```python
from build123d import *

# Parameters (mm, degrees)
EXTRUDE_1_DEPTH     = 3
SKETCH_3_R          = 1.5
CUT_EXTRUDE_1_DEPTH = 3


with BuildPart() as part:
    # 草图2 → 凸台-拉伸1 (new body)
    with BuildSketch(Plane(origin=(0, 0, 0), x_dir=(0, 0, -1), z_dir=(1, 0, 0))):
        with BuildLine():
            Line((0, 0), (0, -15))
            Line((0, -15), (20, -15))
            Line((20, -15), (50, -15))
            Line((50, -15), (70, -15))
            Line((70, -15), (70, 0))
            Line((70, 0), (62.603277808, 0))
            ThreePointArc((62.603277808, 0), (60.294225904, 0.565106619), (58.507118205, 2.132688278))
            Line((58.507118205, 2.132688278), (43.403840397, 23.708799432))
            ThreePointArc((43.403840397, 23.708799432), (42.731310557, 25.07291423), (42.5, 26.576111154))
            Line((42.5, 26.576111154), (42.5, 35))
            Line((42.5, 35), (27.5, 35))
            Line((27.5, 35), (27.5, 26.576111154))
            ThreePointArc((27.5, 26.576111154), (27.268689443, 25.07291423), (26.596159603, 23.708799432))
            Line((26.596159603, 23.708799432), (11.492881795, 2.132688278))
            ThreePointArc((11.492881795, 2.132688278), (9.705774096, 0.565106619), (7.396722192, 0))
            Line((7.396722192, 0), (0, 0))
        make_face()
        with BuildLine():
            Line((22.877485177, -6.367544468), (23.86037961, -3.41886117))
            ThreePointArc((23.86037961, -3.41886117), (25.680244677, -0.943789074), (28.6037961, 0))
            Line((28.6037961, 0), (41.3962039, 0))
            ThreePointArc((41.3962039, 0), (44.319755323, -0.943789074), (46.13962039, -3.41886117))
            Line((46.13962039, -3.41886117), (47.122514823, -6.367544468))
            ThreePointArc((47.122514823, -6.367544468), (46.847632597, -8.169420569), (45.225148227, -9))
            Line((45.225148227, -9), (24.774851773, -9))
            ThreePointArc((24.774851773, -9), (23.152367403, -8.169420569), (22.877485177, -6.367544468))
        make_face(mode=Mode.SUBTRACT)
        with BuildLine():
            Line((29.256242147, 6), (31.5, 6))
            Line((31.5, 6), (31.5, 11))
            ThreePointArc((31.5, 11), (30.914213562, 12.414213562), (29.5, 13))
            Line((29.5, 13), (24.673666452, 13))
            ThreePointArc((24.673666452, 13), (25.072942015, 8.261387212), (29.256242147, 6))
        make_face(mode=Mode.SUBTRACT)
        with BuildLine():
            Line((30.57750685, 21.867311722), (29.256242147, 19))
            Line((29.256242147, 19), (40.091090757, 19))
            Line((40.091090757, 19), (38.769826055, 21.867311722))
            ThreePointArc((38.769826055, 21.867311722), (34.673666452, 24), (30.57750685, 21.867311722))
        make_face(mode=Mode.SUBTRACT)
        with BuildLine():
            Line((38.5, 11), (38.5, 6))
            Line((38.5, 6), (40.091090757, 6))
            ThreePointArc((40.091090757, 6), (44.27439089, 8.261387212), (44.673666452, 13))
            Line((44.673666452, 13), (40.5, 13))
            ThreePointArc((40.5, 13), (39.085786438, 12.414213562), (38.5, 11))
        make_face(mode=Mode.SUBTRACT)
    extrude(amount=EXTRUDE_1_DEPTH)

    # 草图3 → 切除-拉伸1 (cut)
    with BuildSketch(Plane(origin=(3, 0, 0), x_dir=(0, 0, -1), z_dir=(1, 0, 0))):
        with Locations((35, 30)):
            Circle(SKETCH_3_R)
        with Locations((66, -7.5)):
            Circle(SKETCH_3_R)
        with Locations((56, -7.5)):
            Circle(SKETCH_3_R)
        with Locations((14, -7.5)):
            Circle(SKETCH_3_R)
        with Locations((4, -7.5)):
            Circle(SKETCH_3_R)
        with Locations((35, 16)):
            Circle(SKETCH_3_R)
    extrude(amount=-CUT_EXTRUDE_1_DEPTH, mode=Mode.SUBTRACT)


solid = part.part
```
Verification items for the finished model (mm, model axes). A direction names the side the tool comes from. Give positions to 0.01 mm unless a question says otherwise; leave off trailing zeros. Loops run counter-clockwise (first coordinate to the right, second up) from the corner with the lowest first, then second, coordinate; pieces in that order, holes last. Notation, with made-up numbers: M -1.75,83 L 3.25,83 A14 ccw 3.25,99 Z; hole C -15,-31 d9. An arc over 180 degrees is marked long. Return JSON: item names as keys, results as strings.
1) Gauge pin test, flat ends, axial feed: P1, Ø1.5, axis at x = 1, y = 7.5, coming from the +Z side (3 decimals); P2, Ø1.5, axis at x = 1, z = -21.5, coming from the +Y side; P3, Ø1.5, axis at x = 2, y = 9.5, coming from the -Z side (3 decimals). Record the tip position at first contact, or that the pin passes through.
Findings:
{"P1": "stops at z = -14.725", "P2": "stops at y = 17.5", "P3": "stops at z = -53.875"}
2) Mould release check, pull along Y, two halves, no side actions. Record for faces 1 (the flat face through (1, -8, -70)), 2 (the flat face through (1, -9, -35)), 3 (the flat face through (1, 0, -4)), 4 (the cylindrical face through (1.52, -8.83, -4.69)): released by +Y, released by -Y, zero draft, split by the parting line, or undercut.
Findings:
{"face 1": "zero draft", "face 2": "undercut", "face 3": "released by +Y", "face 4": "undercut"}
3) Tool access check on faces 5 (the flat face through (1, 31, -27.5)), 6 (the flat face through (1, 0, -66)), 7 (the cylindrical face through (1.479, -8.191, -23.168)). Record the directions out of +Z, -Z, +X, -X, +Y, -Y that give a thin tool (end or side, any length) a straight path to the whole face; none if there is none.
Findings:
{"face 5": "+Z, +X, -X, +Y", "face 6": "-Z, +X, -X, +Y", "face 7": "+X, -X"}
4) Section check B-B, the plane z = -4. Enter the section's corners in (x, y).
Findings:
{"outline": "M 0,-15 L 3,-15 L 3,-9 L 0,-9 Z; M 0,-6 L 3,-6 L 3,0 L 0,0 Z"}
5) Section check C-C, the plane y = -7.5. Enter the section's corners in (x, z), and give its area (3 significant figures).
Findings:
{"outline": "M 0,-70 L 3,-70 L 3,-67.5 L 0,-67.5 Z; M 0,-64.5 L 3,-64.5 L 3,-57.5 L 0,-57.5 Z; M 0,-54.5 L 3,-54.5 L 3,-47.16 L 0,-47.16 Z; M 0,-22.84 L 3,-22.84 L 3,-15.5 L 0,-15.5 Z; M 0,-12.5 L 3,-12.5 L 3,-5.5 L 0,-5.5 Z; M 0,-2.5 L 3,-2.5 L 3,0 L 0,0 Z", "area": "101 mm2"}
6) Material ranges on L1, parallel to Y at x = 2.3, z = -35; L2, parallel to Y at x = 0.7, z = -32.5; L3, parallel to Z at x = 1.9, y = 9, recorded low to high. Write a range as [from, to].
Findings:
{"L1": "y = [-15, -9], [0, 14.5], [17.5, 19], [23.99, 28.5], [31.5, 35]", "L2": "y = [-15, -9], [0, 19], [23.5, 35]", "L3": "z = [-53.7, -44.67], [-38.5, -31.5], [-24.67, -16.3]"}
7) Section check D-D, the plane z = -35. Enter the section's corners in (x, y), and give its area (3 significant figures).
Findings:
{"outline": "M 0,-15 L 3,-15 L 3,-9 L 0,-9 Z; M 0,0 L 3,0 L 3,14.5 L 0,14.5 Z; M 0,17.5 L 3,17.5 L 3,19 L 0,19 Z; M 0,23.99 L 3,23.99 L 3,28.5 L 0,28.5 Z; M 0,31.5 L 3,31.5 L 3,35 L 0,35 Z", "area": "90.0 mm2"}
8) Section check A-A, the plane y = 16. Enter the section's corners in (x, z), and give its area (3 significant figures).
Findings:
{"outline": "M 0,-48.8 L 3,-48.8 L 3,-36.5 L 0,-36.5 Z; M 0,-33.5 L 3,-33.5 L 3,-21.2 L 0,-21.2 Z", "area": "73.8 mm2"}
